from build123d import *

# Parameters (mm, degrees)
SKETCH1_R           = 1.7
SKETCH1_R_2         = 2.25
BOSS_EXTRUDE1_DEPTH = 1.7
CUT_EXTRUDE1_REACH  = 3.7
SKETCH2_R           = 0.5


with BuildPart() as part:
    # Sketch1 → Boss-Extrude1 (new body)
    with BuildSketch(Plane(origin=(0, 0, 0), x_dir=(1, 0, 0), z_dir=(0, 1, 0))):
        with BuildLine():
            Line((3, 68), (10, 68))
            ThreePointArc((10, 68), (12.121320344, 68.878679656), (13, 71))
            Line((13, 71), (13, 72))
            ThreePointArc((13, 72), (16, 75), (19, 72))
            Line((19, 72), (19, 71))
            ThreePointArc((19, 71), (19.878679656, 68.878679656), (22, 68))
            Line((22, 68), (29, 68))
            ThreePointArc((29, 68), (31.121320344, 67.121320344), (32, 65))
            Line((32, 65), (32, 3))
            ThreePointArc((32, 3), (31.121320344, 0.878679656), (29, 0))
            Line((29, 0), (3, 0))
            ThreePointArc((3, 0), (0.878679656, 0.878679656), (0, 3))
            Line((0, 3), (0, 65))
            ThreePointArc((0, 65), (0.878679656, 67.121320344), (3, 68))
        make_face()
        with Locations((16, 72)):
            Circle(SKETCH1_R, mode=Mode.SUBTRACT)
        with Locations((29, 3)):
            Circle(SKETCH1_R, mode=Mode.SUBTRACT)
        with Locations((3, 3)):
            Circle(SKETCH1_R, mode=Mode.SUBTRACT)
        with Locations((16, 65)):
            Circle(SKETCH1_R_2, mode=Mode.SUBTRACT)
    extrude(amount=BOSS_EXTRUDE1_DEPTH)

    # Sketch2 → Cut-Extrude1 (cut, up to next)
    with BuildSketch(Plane(origin=(0, 1.7, 0), x_dir=(1, 0, 0), z_dir=(0, 1, 0)), mode=Mode.PRIVATE) as cut_extrude1_sk1:
        with Locations((8, 1.9)):
            Circle(SKETCH2_R)
    cut_extrude1_tool1 = extrude(cut_extrude1_sk1.sketch, amount=-CUT_EXTRUDE1_REACH, mode=Mode.PRIVATE) & part.part
    add(cut_extrude1_tool1.solids().sort_by_distance((8, 1.7, -1.9))[0], mode=Mode.SUBTRACT)
    # Sketch2 → Cut-Extrude1 (cut, up to next)
    with BuildSketch(Plane(origin=(0, 1.7, 0), x_dir=(1, 0, 0), z_dir=(0, 1, 0)), mode=Mode.PRIVATE) as cut_extrude1_sk2:
        with Locations((8, 4.44)):
            Circle(SKETCH2_R)
    cut_extrude1_tool2 = extrude(cut_extrude1_sk2.sketch, amount=-CUT_EXTRUDE1_REACH, mode=Mode.PRIVATE) & part.part
    add(cut_extrude1_tool2.solids().sort_by_distance((8, 1.7, -4.44))[0], mode=Mode.SUBTRACT)
    # Sketch2 → Cut-Extrude1 (cut, up to next)
    with BuildSketch(Plane(origin=(0, 1.7, 0), x_dir=(1, 0, 0), z_dir=(0, 1, 0)), mode=Mode.PRIVATE) as cut_extrude1_sk3:
        with Locations((8, 6.98)):
            Circle(SKETCH2_R)
    cut_extrude1_tool3 = extrude(cut_extrude1_sk3.sketch, amount=-CUT_EXTRUDE1_REACH, mode=Mode.PRIVATE) & part.part
    add(cut_extrude1_tool3.solids().sort_by_distance((8, 1.7, -6.98))[0], mode=Mode.SUBTRACT)
    # Sketch2 → Cut-Extrude1 (cut, up to next)
    with BuildSketch(Plane(origin=(0, 1.7, 0), x_dir=(1, 0, 0), z_dir=(0, 1, 0)), mode=Mode.PRIVATE) as cut_extrude1_sk4:
        with Locations((24, 6.98)):
            Circle(SKETCH2_R)
    cut_extrude1_tool4 = extrude(cut_extrude1_sk4.sketch, amount=-CUT_EXTRUDE1_REACH, mode=Mode.PRIVATE) & part.part
    add(cut_extrude1_tool4.solids().sort_by_distance((24, 1.7, -6.98))[0], mode=Mode.SUBTRACT)
    # Sketch2 → Cut-Extrude1 (cut, up to next)
    with BuildSketch(Plane(origin=(0, 1.7, 0), x_dir=(1, 0, 0), z_dir=(0, 1, 0)), mode=Mode.PRIVATE) as cut_extrude1_sk5:
        with Locations((24, 4.44)):
            Circle(SKETCH2_R)
    cut_extrude1_tool5 = extrude(cut_extrude1_sk5.sketch, amount=-CUT_EXTRUDE1_REACH, mode=Mode.PRIVATE) & part.part
    add(cut_extrude1_tool5.solids().sort_by_distance((24, 1.7, -4.44))[0], mode=Mode.SUBTRACT)
    # Sketch2 → Cut-Extrude1 (cut, up to next)
    with BuildSketch(Plane(origin=(0, 1.7, 0), x_dir=(1, 0, 0), z_dir=(0, 1, 0)), mode=Mode.PRIVATE) as cut_extrude1_sk6:
        with Locations((24, 1.9)):
            Circle(SKETCH2_R)
    cut_extrude1_tool6 = extrude(cut_extrude1_sk6.sketch, amount=-CUT_EXTRUDE1_REACH, mode=Mode.PRIVATE) & part.part
    add(cut_extrude1_tool6.solids().sort_by_distance((24, 1.7, -1.9))[0], mode=Mode.SUBTRACT)
    # Sketch2 → Cut-Extrude1 (cut, up to next)
    with BuildSketch(Plane(origin=(0, 1.7, 0), x_dir=(1, 0, 0), z_dir=(0, 1, 0)), mode=Mode.PRIVATE) as cut_extrude1_sk7:
        with Locations((7.11, 10)):
            Circle(SKETCH2_R)
    cut_extrude1_tool7 = extrude(cut_extrude1_sk7.sketch, amount=-CUT_EXTRUDE1_REACH, mode=Mode.PRIVATE) & part.part
    add(cut_extrude1_tool7.solids().sort_by_distance((7.11, 1.7, -10))[0], mode=Mode.SUBTRACT)
    # Sketch2 → Cut-Extrude1 (cut, up to next)
    with BuildSketch(Plane(origin=(0, 1.7, 0), x_dir=(1, 0, 0), z_dir=(0, 1, 0)), mode=Mode.PRIVATE) as cut_extrude1_sk8:
        with Locations((9.65, 10)):
            Circle(SKETCH2_R)
    cut_extrude1_tool8 = extrude(cut_extrude1_sk8.sketch, amount=-CUT_EXTRUDE1_REACH, mode=Mode.PRIVATE) & part.part
    add(cut_extrude1_tool8.solids().sort_by_distance((9.65, 1.7, -10))[0], mode=Mode.SUBTRACT)
    # Sketch2 → Cut-Extrude1 (cut, up to next)
    with BuildSketch(Plane(origin=(0, 1.7, 0), x_dir=(1, 0, 0), z_dir=(0, 1, 0)), mode=Mode.PRIVATE) as cut_extrude1_sk9:
        with Locations((12.19, 10)):
            Circle(SKETCH2_R)
    cut_extrude1_tool9 = extrude(cut_extrude1_sk9.sketch, amount=-CUT_EXTRUDE1_REACH, mode=Mode.PRIVATE) & part.part
    add(cut_extrude1_tool9.solids().sort_by_distance((12.19, 1.7, -10))[0], mode=Mode.SUBTRACT)
    # Sketch2 → Cut-Extrude1 (cut, up to next)
    with BuildSketch(Plane(origin=(0, 1.7, 0), x_dir=(1, 0, 0), z_dir=(0, 1, 0)), mode=Mode.PRIVATE) as cut_extrude1_sk10:
        with Locations((14.73, 10)):
            Circle(SKETCH2_R)
    cut_extrude1_tool10 = extrude(cut_extrude1_sk10.sketch, amount=-CUT_EXTRUDE1_REACH, mode=Mode.PRIVATE) & part.part
    add(cut_extrude1_tool10.solids().sort_by_distance((14.73, 1.7, -10))[0], mode=Mode.SUBTRACT)
    # Sketch2 → Cut-Extrude1 (cut, up to next)
    with BuildSketch(Plane(origin=(0, 1.7, 0), x_dir=(1, 0, 0), z_dir=(0, 1, 0)), mode=Mode.PRIVATE) as cut_extrude1_sk11:
        with Locations((17.27, 10)):
            Circle(SKETCH2_R)
    cut_extrude1_tool11 = extrude(cut_extrude1_sk11.sketch, amount=-CUT_EXTRUDE1_REACH, mode=Mode.PRIVATE) & part.part
    add(cut_extrude1_tool11.solids().sort_by_distance((17.27, 1.7, -10))[0], mode=Mode.SUBTRACT)
    # Sketch2 → Cut-Extrude1 (cut, up to next)
    with BuildSketch(Plane(origin=(0, 1.7, 0), x_dir=(1, 0, 0), z_dir=(0, 1, 0)), mode=Mode.PRIVATE) as cut_extrude1_sk12:
        with Locations((19.81, 10)):
            Circle(SKETCH2_R)
    cut_extrude1_tool12 = extrude(cut_extrude1_sk12.sketch, amount=-CUT_EXTRUDE1_REACH, mode=Mode.PRIVATE) & part.part
    add(cut_extrude1_tool12.solids().sort_by_distance((19.81, 1.7, -10))[0], mode=Mode.SUBTRACT)
    # Sketch2 → Cut-Extrude1 (cut, up to next)
    with BuildSketch(Plane(origin=(0, 1.7, 0), x_dir=(1, 0, 0), z_dir=(0, 1, 0)), mode=Mode.PRIVATE) as cut_extrude1_sk13:
        with Locations((22.35, 10)):
            Circle(SKETCH2_R)
    cut_extrude1_tool13 = extrude(cut_extrude1_sk13.sketch, amount=-CUT_EXTRUDE1_REACH, mode=Mode.PRIVATE) & part.part
    add(cut_extrude1_tool13.solids().sort_by_distance((22.35, 1.7, -10))[0], mode=Mode.SUBTRACT)
    # Sketch2 → Cut-Extrude1 (cut, up to next)
    with BuildSketch(Plane(origin=(0, 1.7, 0), x_dir=(1, 0, 0), z_dir=(0, 1, 0)), mode=Mode.PRIVATE) as cut_extrude1_sk14:
        with Locations((24.89, 10)):
            Circle(SKETCH2_R)
    cut_extrude1_tool14 = extrude(cut_extrude1_sk14.sketch, amount=-CUT_EXTRUDE1_REACH, mode=Mode.PRIVATE) & part.part
    add(cut_extrude1_tool14.solids().sort_by_distance((24.89, 1.7, -10))[0], mode=Mode.SUBTRACT)
    # Sketch2 → Cut-Extrude1 (cut, up to next)
    with BuildSketch(Plane(origin=(0, 1.7, 0), x_dir=(1, 0, 0), z_dir=(0, 1, 0)), mode=Mode.PRIVATE) as cut_extrude1_sk15:
        with Locations((9.65, 12.54)):
            Circle(SKETCH2_R)
    cut_extrude1_tool15 = extrude(cut_extrude1_sk15.sketch, amount=-CUT_EXTRUDE1_REACH, mode=Mode.PRIVATE) & part.part
    add(cut_extrude1_tool15.solids().sort_by_distance((9.65, 1.7, -12.54))[0], mode=Mode.SUBTRACT)
    # Sketch2 → Cut-Extrude1 (cut, up to next)
    with BuildSketch(Plane(origin=(0, 1.7, 0), x_dir=(1, 0, 0), z_dir=(0, 1, 0)), mode=Mode.PRIVATE) as cut_extrude1_sk16:
        with Locations((12.19, 12.54)):
            Circle(SKETCH2_R)
    cut_extrude1_tool16 = extrude(cut_extrude1_sk16.sketch, amount=-CUT_EXTRUDE1_REACH, mode=Mode.PRIVATE) & part.part
    add(cut_extrude1_tool16.solids().sort_by_distance((12.19, 1.7, -12.54))[0], mode=Mode.SUBTRACT)
    # Sketch2 → Cut-Extrude1 (cut, up to next)
    with BuildSketch(Plane(origin=(0, 1.7, 0), x_dir=(1, 0, 0), z_dir=(0, 1, 0)), mode=Mode.PRIVATE) as cut_extrude1_sk17:
        with Locations((14.73, 12.54)):
            Circle(SKETCH2_R)
    cut_extrude1_tool17 = extrude(cut_extrude1_sk17.sketch, amount=-CUT_EXTRUDE1_REACH, mode=Mode.PRIVATE) & part.part
    add(cut_extrude1_tool17.solids().sort_by_distance((14.73, 1.7, -12.54))[0], mode=Mode.SUBTRACT)
    # Sketch2 → Cut-Extrude1 (cut, up to next)
    with BuildSketch(Plane(origin=(0, 1.7, 0), x_dir=(1, 0, 0), z_dir=(0, 1, 0)), mode=Mode.PRIVATE) as cut_extrude1_sk18:
        with Locations((17.27, 12.54)):
            Circle(SKETCH2_R)
    cut_extrude1_tool18 = extrude(cut_extrude1_sk18.sketch, amount=-CUT_EXTRUDE1_REACH, mode=Mode.PRIVATE) & part.part
    add(cut_extrude1_tool18.solids().sort_by_distance((17.27, 1.7, -12.54))[0], mode=Mode.SUBTRACT)
    # Sketch2 → Cut-Extrude1 (cut, up to next)
    with BuildSketch(Plane(origin=(0, 1.7, 0), x_dir=(1, 0, 0), z_dir=(0, 1, 0)), mode=Mode.PRIVATE) as cut_extrude1_sk19:
        with Locations((19.81, 12.54)):
            Circle(SKETCH2_R)
    cut_extrude1_tool19 = extrude(cut_extrude1_sk19.sketch, amount=-CUT_EXTRUDE1_REACH, mode=Mode.PRIVATE) & part.part
    add(cut_extrude1_tool19.solids().sort_by_distance((19.81, 1.7, -12.54))[0], mode=Mode.SUBTRACT)
    # Sketch2 → Cut-Extrude1 (cut, up to next)
    with BuildSketch(Plane(origin=(0, 1.7, 0), x_dir=(1, 0, 0), z_dir=(0, 1, 0)), mode=Mode.PRIVATE) as cut_extrude1_sk20:
        with Locations((22.35, 12.54)):
            Circle(SKETCH2_R)
    cut_extrude1_tool20 = extrude(cut_extrude1_sk20.sketch, amount=-CUT_EXTRUDE1_REACH, mode=Mode.PRIVATE) & part.part
    add(cut_extrude1_tool20.solids().sort_by_distance((22.35, 1.7, -12.54))[0], mode=Mode.SUBTRACT)
    # Sketch2 → Cut-Extrude1 (cut, up to next)
    with BuildSketch(Plane(origin=(0, 1.7, 0), x_dir=(1, 0, 0), z_dir=(0, 1, 0)), mode=Mode.PRIVATE) as cut_extrude1_sk21:
        with Locations((24.89, 12.54)):
            Circle(SKETCH2_R)
    cut_extrude1_tool21 = extrude(cut_extrude1_sk21.sketch, amount=-CUT_EXTRUDE1_REACH, mode=Mode.PRIVATE) & part.part
    add(cut_extrude1_tool21.solids().sort_by_distance((24.89, 1.7, -12.54))[0], mode=Mode.SUBTRACT)
    # Sketch2 → Cut-Extrude1 (cut, up to next)
    with BuildSketch(Plane(origin=(0, 1.7, 0), x_dir=(1, 0, 0), z_dir=(0, 1, 0)), mode=Mode.PRIVATE) as cut_extrude1_sk22:
        with Locations((7.11, 12.54)):
            Circle(SKETCH2_R)
    cut_extrude1_tool22 = extrude(cut_extrude1_sk22.sketch, amount=-CUT_EXTRUDE1_REACH, mode=Mode.PRIVATE) & part.part
    add(cut_extrude1_tool22.solids().sort_by_distance((7.11, 1.7, -12.54))[0], mode=Mode.SUBTRACT)


solid = part.part
Design review of the part built by this model. Coordinates are the model's own, in mm. A direction names the side the tool comes from. Coordinates: 2 decimals unless noted, no trailing zeros. Loops run counter-clockwise (first coordinate to the right, second up) from the corner with the lowest first, then second, coordinate; pieces in that order, holes last. Notation, with made-up numbers: (61, 74.25) -> (67, 74.25) arc R19 ccw to (67, 97.25) -> close; hole circle Ø9 at (32, 83.25). An arc over 180 degrees is marked (long way). Use a Markdown table: item, result. Add a question column.
Item 1: Wall thickness on L1, parallel to X at y = 0.95, z = -3; L2, parallel to X at y = 0.75, z = -6.98; L3, parallel to Z at x = 22.35, y = 0.7: over which ranges is each line inside the solid? List them lowest first. Write a range as from..to.
Item 2: We need section A-A, the plane x = 16. Write out the cut boundary in (y, z).
Item 3: We need section B-B, the plane y = 1.35. Count the separate pieces of the cut face and the enclosed holes in it, and give its area (3 significant figures).
Item 4: The part is to be moulded in two halves that separate along Z. For faces 1 (the cylindrical face through (19.86, 0.84, -68.9)), 2 (the cylindrical face through (16.8, 0.8, -70.5)), 3 (the flat face through (32, 1, -34)), say which applies: +Z half, -Z half, draft (parallel to the pull), parting line (faces both ways), or undercut.
Item 5: Machinability: for faces 4 (the flat face through (25, 1, -68)), 5 (the flat face through (0, 1, -34)), 6 (the flat face through (6, 1, -68)), which of the approach directions +Z, -Z, +X, -X, +Y, -Y give a long, thin tool a straight path to every point of the face, cutting with its end or side? Answer none if there is none.
Item 6: Clearance check with flat-ended pins moving along their axes: P1, Ø2.5, axis at x = 16, z = -65, coming from the -Y side; P2, Ø0.8, axis at x = 25, y = 1, coming from the -Z side; P3, Ø4, axis at x = 16, z = -72, coming from the -Y side; P4, Ø0.5, axis at y = 1.5, z = -71.5, coming from the +X side. State where each tip first meets the part, or that it passes through.
Numbers:
| question | item | result |
|---|---|---|
| 1 | L1 | x = 0..1.3, 4.7..27.3, 30.7..32 |
| 1 | L2 | x = 0..7.5, 8.5..23.5, 24.5..32 |
| 1 | L3 | z = -68..-13.04, -12.04..-10.5, -9.5..0 |
| 2 | outline | (0, -75) -> (1.7, -75) -> (1.7, -73.7) -> (0, -73.7) -> close; (0, -70.3) -> (1.7, -70.3) -> (1.7, -67.25) -> (0, -67.25) -> close; (0, -62.75) -> (1.7, -62.75) -> (1.7, 0) -> (0, 0) -> close |
| 3 | separate pieces | 1 |
| 3 | enclosed holes | 26 |
| 3 | area | 2,150 mm^2 |
| 4 | face 1 | -Z half |
| 4 | face 2 | undercut |
| 4 | face 3 | draft |
| 5 | face 4 | -Z, +X, +Y, -Y |
| 5 | face 5 | +Z, -Z, -X, +Y, -Y |
| 5 | face 6 | -Z, -X, +Y, -Y |
| 6 | P1 | passes through |
| 6 | P2 | stops at z = -68 |
| 6 | P3 | stops at y = 0 |
| 6 | P4 | stops at x = 19 |
